from build123d import *

# Parameters (mm, degrees)
SKETCH1_R           = 1.5
BOSS_EXTRUDE4_DEPTH = 4
SKETCH2_R           = 3
BOSS_EXTRUDE6_DEPTH = 4
CUT_EXTRUDE4_DEPTH  = 5.0000001
FILLET4_R           = 2
SKETCH7_R           = 5
SKETCH7_R_2         = 1.5
CUT_EXTRUDE3_DEPTH  = 10


with BuildPart() as part:
    # Sketch1 → Boss-Extrude4 (new body)
    with BuildSketch(Plane(origin=(0, 0, 0), x_dir=(1, 0, 0), z_dir=(0, 1, 0))):
        with BuildLine():
            add(Edge.make_bspline(
                [(0, 15), (-53.333333333, 15), (-97.583223813, -2.850327116), (-150.232513174, -43.74649777)],
                knots=[0, 0, 0, 0, 1, 1, 1, 1], degree=3))
            Line((-150.232513174, -43.74649777), (-144.167389057, -51.554673195))
            add(Edge.make_bspline(
                [(0, -15), (-49.211171611, -15), (-112.57781544, -27.016970802), (-144.167389057, -51.554673195)],
                knots=[0, 0, 0, 0, 1, 1, 1, 1], degree=3))
            ThreePointArc((0, -15), (15, 0), (0, 15))
        make_face()
        with Locations((-143.201136916, -44.647893409)):
            Circle(SKETCH1_R, mode=Mode.SUBTRACT)
    extrude(amount=BOSS_EXTRUDE4_DEPTH)

    # Sketch2 → Boss-Extrude6 (add)
    with BuildSketch(Plane.XZ):
        with BuildLine():
            Line((24.745562632, -11.732737533), (12.800284575, 7.820020128))
            ThreePointArc((12.800284575, 7.820020128), (14.439602983, 4.061756478), (15, 0))
            ThreePointArc((15, 0), (10.606601718, -10.606601718), (0, -15))
            add(Edge.make_bspline(
                [(0, -15), (-9.352958156, -15), (-18.426564807, -14.451032409), (-27.315109341, -13.325076493)],
                knots=[0, 0, 0, 0, 0.175367965, 0.175367965, 0.175367965, 0.175367965], degree=3))
            Line((-27.315109341, -13.325076493), (19.850447753, -19.299770983))
            ThreePointArc((19.850447753, -19.299770983), (24.676955739, -17.055197662), (24.745562632, -11.732737533))
        make_face()
        with Locations((20.478801107, -14.339410909)):
            Circle(SKETCH2_R, mode=Mode.SUBTRACT)
    extrude(amount=-BOSS_EXTRUDE6_DEPTH)

    # Sketch8 → Cut-Extrude4 (cut, through all)
    with BuildSketch(Plane(origin=(0, 4, 0), x_dir=(1, 0, 0), z_dir=(0, 1, 0))):
        Polygon((-61.93012476, 5.733160203), (-24.428772421, -15.918255665), (-81.418617577, -101.346773657), (-136.224202564, -112.686812452), (-181.390604498, 23.006558879), align=None)
    extrude(amount=-CUT_EXTRUDE4_DEPTH, mode=Mode.SUBTRACT)

    # Fillet4
    fillet4_edges = [part.edges().sort_by_distance(p)[0] for p in [
        (-61.93012476, 2, -5.733160203),
        (-24.428772421, 2, 15.918255665),
    ]]
    fillet(fillet4_edges, radius=FILLET4_R)

    # Sketch7 → Cut-Extrude3 (cut)
    with BuildSketch(Plane(origin=(0, 4, 0), x_dir=(1, 0, 0), z_dir=(0, 1, 0))):
        Circle(SKETCH7_R)
        with Locations((-42.326653454, 1.343293998)):
            Circle(SKETCH7_R_2)
        with Locations((-20.67601836, -11.156706002)):
            Circle(SKETCH7_R_2)
        with Locations((-20.67601836, 1.343293998)):
            Circle(SKETCH7_R_2)
    extrude(amount=-CUT_EXTRUDE3_DEPTH, mode=Mode.SUBTRACT)


solid = part.part
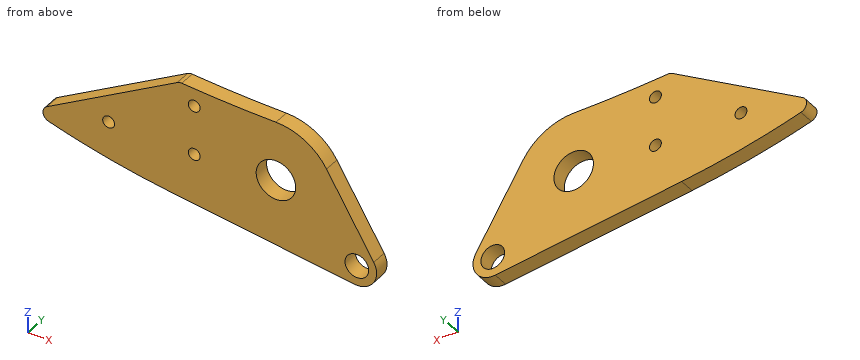
Could you check a few things on this model? Use its own coordinates, in mm. Give positions to 0.01 mm unless a question says otherwise; leave off trailing zeros.
1. Suppose I cut it at A-A (y = 1.75). Give the number of separate pieces and of enclosed holes in the cut face, plus the area to 3 significant figures.
2. Will these pins go through, and if not, where does the flat tip stop? P1, Ø3.5, axis at x = -20.68, z = -1.34, coming from the +Y side; P2, Ø2.5, axis at x = -20.68, z = 11.16, coming from the +Y side.
3. I need wall thicknesses on L1, parallel to X at y = 3.7, z = -1; L2, parallel to X at y = 3.55, z = 0; L3, parallel to X at y = 3.8, z = 4.5. Which ranges of each line are inside material? Lowest first, please.
Solved:
1. separate pieces: 1
1. enclosed holes: 5
1. area: 1,790 mm2
2. P1: stops at y = 4
2. P2: passes through
3. L1: x = -53.73 to -43.79, -40.87 to -22.14, -19.22 to -4.9, 4.9 to 18.19
3. L2: x = -52 to -42.99, -41.66 to -21.34, -20.01 to -5, 5 to 17.58
3. L3: x = -44.21 to -2.18, 2.18 to 14.83
